Could you check a few things on this model? Use its own coordinates, in mm. Face numbers are marked on the shaded views. A direction names the side the tool comes from. Coordinates: 2 decimals unless noted, no trailing zeros. Loops run counter-clockwise (first coordinate to the right, second up) from the corner with the lowest first, then second, coordinate; pieces in that order, holes last. Notation, with made-up numbers: (-15, 79) -> (39, 79) arc R13 cw to (39, 94) -> close; hole circle Ø6 at (-15, 25.5). An arc over 180 degrees is marked (long way). One line per question, with ' | ' between items. Start each with the question number.
(1) Suppose I cut it at A-A (z = -15.75). Please give me the cut outline in (x, y), plus the area to 3 significant figures.
(2) If I drill on line 1 along X through (y, z) = (5.75, -19.5), over which ranges is the centre line in solid material (lowest first)?
(3) Which directions (+Z, -Z, +X, -X, +Y, -Y) give clear straight access to the entire face, cutting with the end or side of a thin tool? Please do the marked faces 1 and 2.
(4) I'm going to push flat-ended pins straight in: pin 1 Ø5 at (y, z) = (-2, -3.5) entering from +X; pin 2 Ø0.5 at (x, y) = (33, -14.5) entering from +Z; pin 3 Ø0.8 at (x, y) = (-32, -14.5) entering from -Z. Where does each tip first touch, or does it pass through?
(5) Suppose I cut it at B-B (y = -0.75). Please give me the cut outline in (x, z), plus the area to 3 significant figures.
(6) Suppose I cut it at C-C (z = -6.5). Please give me the cut outline in (x, y), plus the area to 3 significant figures.
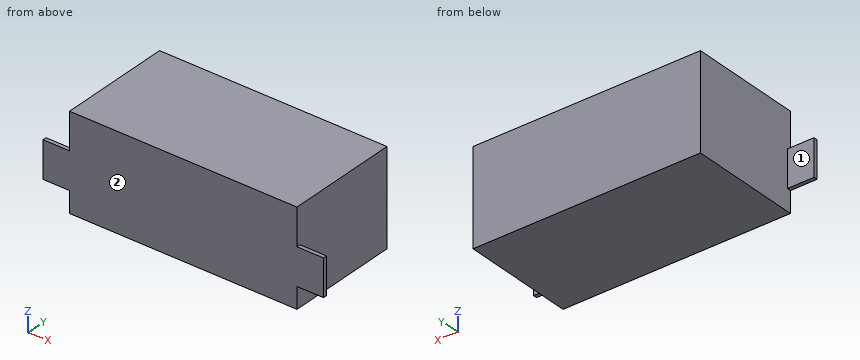
Autodesk Inventor part; units mm, degrees
ref_plane "YZ Plane" through (0, 0, 0) normal (1, 0, 0) x (0, 1, 0)
ref_plane "XZ Plane" through (0, 0, 0) normal (0, 1, 0) x (-1, 0, 0)
ref_plane "XY Plane" through (0, 0, 0) normal (0, 0, 1) x (1, 0, 0)
sketch "Skizze1" plane through (0, 0, 0) normal (0, 0, 1) x (1, 0, 0)
  line L0 (30, -15) -> (-30, -15)
  line L1 (-30, -15) -> (-30, 15)
  line L2 (-30, 15) -> (30, 15)
  line L3 (30, 15) -> (30, -15)
  point P0 (0, 0)
  point P1 (-30, 0)
  point P2 (0, 15)
  dimension "d0" = 30
  dimension "d1" = 60
extrude "Extrusion1" add sketch "Skizze1" against normal blind 25
sketch "Skizze4" plane through (30, -15, 0) normal (1, 0, 0) x (0, 0, -1)
  line L0 (0, 0) -> (0, 30)
  line L1 (0, 0) -> (25, 0)
  line L2 (25, 0) -> (19.4, 0)
  line L3 (9.7, 0) -> (19.4, 0)
  line L4 (19.4, 0) -> (19.4, 1)
  line L5 (19.4, 1) -> (9.7, 1)
  line L6 (9.7, 1) -> (9.7, 0)
  point P0 (0, 15)
extrude "Extrusion3" add sketch "Skizze4" along normal blind 7
mirror "Spiegeln1" about plane through (0, 0, 0) normal (1, 0, 0) of "Extrusion3"
sketch "Skizze5" plane through (30, -14, -9.7) normal (0, 1, 0) x (1, 0, 0)
  line L0 (7, 0) -> (7, 9.7)
  line L1 (0, -9.7) -> (0, 15.3)
  line L2 (0, -9.7) -> (0, 0)
  line L3 (-60, 9.7) -> (-60, 0)
  line L4 (-60, 9.7) -> (-67, 9.7)
  line L5 (-67, 9.7) -> (-67, 0)
  point P0 (-30, -9.7)
  point P1 (3.5, 4.7412)
  point P2 (-63.5, 4.85)
sketch "Skizze6" plane through (-30, 15, 0) normal (0, 1, 0) x (1, 0, 0)
  line L0 (18.8891, 23.5916) -> (66.0849, 23.5916) construction
  line L1 (66.0849, 23.5916) -> (66.0849, 19.2386) construction
  line L2 (66.0849, 19.2386) -> (18.8891, 19.2386) construction
  line L3 (18.8891, 19.2386) -> (18.8891, 23.5916) construction
  point P0 (30, 0)
properties part number "Empfänger" material "Gold"
Checks:
1) outline: (-37, -15) -> (37, -15) -> (37, -14) -> (30, -14) -> (30, 15) -> (-30, 15) -> (-30, -14) -> (-37, -14) -> close | area: 1,810 mm^2
2) line 1: x = -30 to 30
3) face 1: +Z, -Z, -X, +Y | face 2: +Z, -Z, +X, -X, -Y
4) pin 1: stops at x = 30 | pin 2: stops at z = -9.7 | pin 3: stops at z = -19.4
5) outline: (-30, -25) -> (30, -25) -> (30, 0) -> (-30, 0) -> close | area: 1,500 mm^2
6) outline: (-30, -15) -> (30, -15) -> (30, 15) -> (-30, 15) -> close | area: 1,800 mm^2
